For this review, take the finished solid that the model builds, in its own axes (mm). A direction names the side the tool comes from. Coordinates: 2 decimals unless noted, no trailing zeros. Answer as a JSON object with one key per item and string values. Group by question number.
Item 1: Clearance check with a flat-ended pin moving along its axis: pin 1 (6.5 mm diameter, centred on y = 23.5, z = 49.5, fed in from -X). State where the tip first meets the part, or that it passes through.
Item 2: Mouldability with a two-part tool opening along Y and no side actions: class faces 1 (the flat face through (18.415, 22, 1)), 2 (the flat face through (3.131, 20.262, 54.828)), 3 (the flat face through (9, 44.069, 1)) as released by +Y, released by -Y, zero draft, split by the parting line, or undercut.
Item 3: We need section A-A (x = 3). State how many separate pieces and enclosed holes the cut face has, then the cut area to 3 significant figures.
Item 4: To check wall thickness, follow line 1 (Z direction, x = 12.25, y = 23.5); line 2 (Y direction, x = 5.25, z = 53.5); line 3 (Y direction, x = 0.5, z = 50.5). State the ranges of each line that lie inside material, in increasing order.
Item 5: Tool access review of faces 4 (the flat face through (9, 22, -76.2)), 5 (the flat face through (12.7, 33, 53)): name each direction out of +Z, -Z, +X, -X, +Y, -Y from which nothing blocks a thin tool from reaching the whole face with its end or side.
from build123d import *

# Parameters (mm, degrees)
SKETCH1_W           = 18.415
SKETCH1_H           = 44.069
BOSS_EXTRUDE1_DEPTH = 76.2
SKETCH2_R           = 9.9187
CUT_EXTRUDE1_DEPTH  = 12.7
SKETCH3_R           = 9.525
BOSS_EXTRUDE2_DEPTH = 12.7
CUT_EXTRUDE2_DEPTH  = 6.35
CHAMFER1_SIZE       = 0.635


with BuildPart() as part:
    # Sketch1 → Boss-Extrude1 (new, symmetric)
    with BuildSketch(Plane.XY):
        with Locations((9.2075, 22.0345)):
            Rectangle(SKETCH1_W, SKETCH1_H)
    extrude(amount=BOSS_EXTRUDE1_DEPTH, both=True)

    # Sketch2 → Cut-Extrude1 (cut)
    with BuildSketch(Plane(origin=(0, 0, 0), x_dir=(0, 0, -1), z_dir=(1, 0, 0))):
        with Locations((-49.6062, 23.876)):
            Circle(SKETCH2_R)
        with Locations((49.6062, 23.876)):
            Circle(SKETCH2_R)
    extrude(amount=CUT_EXTRUDE1_DEPTH, mode=Mode.SUBTRACT)

    # Sketch3 → Boss-Extrude2 (add)
    with BuildSketch(Plane.ZY.offset(-12.7)):
        with Locations(Location((49.6062, 23.876, 0), (0, 0, 180))):
            Circle(SKETCH3_R)
        with Locations(Location((-49.6062, 23.876, 0), (0, 0, 180))):
            Circle(SKETCH3_R)
    extrude(amount=BOSS_EXTRUDE2_DEPTH)

    # Sketch4 → Cut-Extrude2 (cut)
    with BuildSketch(Plane.ZY):
        Polygon((42.293794683, 24.416427442), (45.481973448, 17.813484954), (52.794378764, 17.273057512), (56.918605317, 23.335572558), (53.730426552, 29.938515046), (46.418021236, 30.478942488), align=None)
        Polygon((-42.293794683, 24.416427442), (-46.418021236, 30.478942488), (-53.730426552, 29.938515046), (-56.918605317, 23.335572558), (-52.794378764, 17.273057512), (-45.481973448, 17.813484954), align=None)
    extrude(amount=-CUT_EXTRUDE2_DEPTH, mode=Mode.SUBTRACT)

    # Chamfer1
    chamfer1_edges = [part.edges().sort_by_distance(p)[0] for p in [
        (0, 23.876, 59.1312),
        (0, 23.876, -40.0812),
    ]]
    chamfer(chamfer1_edges, length=CHAMFER1_SIZE)


solid = part.part
Check sheet entries:
{
 "1": {"pin 1": "stops at x = 6.35"},
 "2": {"face 1": "zero draft", "face 2": "undercut", "face 3": "released by +Y"},
 "3": {"separate pieces": "3", "enclosed holes": "4", "area": "6,390 mm2"},
 "4": {"line 1": "z = -76.2 to -59.52, -59.12 to -40.09, -39.69 to 39.69, 40.09 to 59.12, 59.52 to 76.2", "line 2": "y = 0 to 14.75, 15.18 to 18.31, 29.96 to 32.57, 33 to 44.07", "line 3": "y = 0 to 14, 14.53 to 17.44, 30.18 to 33.22, 33.75 to 44.07"},
 "5": {"face 4": "-Z, +X, -X, +Y, -Y", "face 5": "-X"}
}
